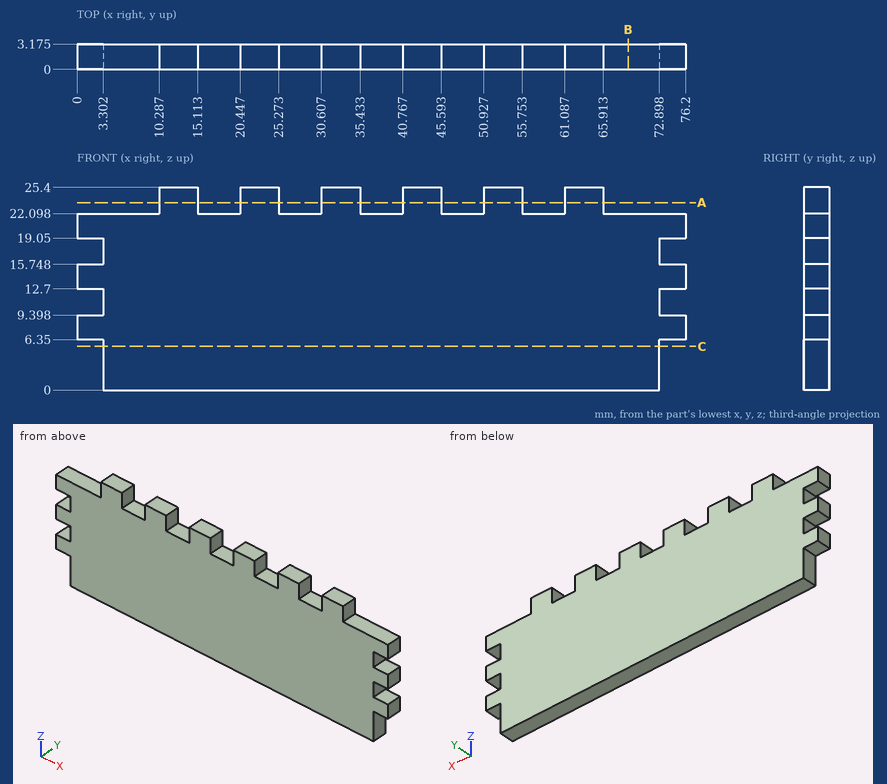
Here's the drawing with two shaded views (mm, measured from the low corner). I have some questions. Coordinates: 2 decimals unless noted, no trailing zeros. Order: outer loops, then holes, each group sorted by start corner. A loop starts at its lowest first (then second) coordinate and runs counter-clockwise, first axis right, second up. Notation, with made-up numbers: M 30,69 L 48,69 A37 ccw 48,105 Z; hole C 79,22 d11. An arc over 180 degrees is marked long. Write item = value, one per line.
(1) For pin 1 Ø1.6 at (y, z) = (1.5, 4) entering from -X; pin 2 Ø1 at (y, z) = (2, 23) entering from +X; pin 3 Ø1 at (x, y) = (74.5, 1) entering from -Z, each with a flat end and sliding along its axis, tell me the tip position at first contact or that it passes through.
Results are:
pin_1 = 3.3
pin_2 = 65.91
pin_3 = 6.35
(2) Suppose I cut it at C-C on z = 5.5. Please give me the cut outline in (x, y) (3 decimals).
Results are:
outline = M 3.302,0 L 72.898,0 L 72.898,3.175 L 3.302,3.175 Z
(3) Suppose I cut it at A-A on z = 23.5. Please give me the cut outline in (x, y) (3 decimals), plus the area to 3 significant figures.
Results are:
outline = M 10.287,0 L 15.113,0 L 15.113,3.175 L 10.287,3.175 Z; M 20.447,0 L 25.273,0 L 25.273,3.175 L 20.447,3.175 Z; M 30.607,0 L 35.433,0 L 35.433,3.175 L 30.607,3.175 Z; M 40.767,0 L 45.593,0 L 45.593,3.175 L 40.767,3.175 Z; M 50.927,0 L 55.753,0 L 55.753,3.175 L 50.927,3.175 Z; M 61.087,0 L 65.913,0 L 65.913,3.175 L 61.087,3.175 Z
area = 91.9 mm2
(4) Suppose I cut it at B-B on x = 69. Please give me the cut outline in (y, z) (3 decimals), plus the area to 3 significant figures.
Results are:
outline = M 0,0 L 3.175,0 L 3.175,22.098 L 0,22.098 Z
area = 70.2 mm2
(5) I need wall thicknesses on line 1 along X through (y, z) = (1.4, 23.25); line 2 along X through (y, z) = (0.75, 16.25); line 3 along Z through (x, y) = (60, 2.15). Which ranges of each line are inside material? Lowest first, please. Write a range as [from, to].
Results are:
line_1 = [10.29, 15.11], [20.45, 25.27], [30.61, 35.43], [40.77, 45.59], [50.93, 55.75], [61.09, 65.91]
line_2 = [3.3, 72.9]
line_3 = [0, 22.1]
